The listing builds one solid part. Answer for the finished solid, in the listing's coordinates (mm). A direction names the side the tool comes from. Coordinates: 2 decimals unless noted, no trailing zeros. Loops run counter-clockwise (first coordinate to the right, second up) from the corner with the lowest first, then second, coordinate; pieces in that order, holes last. Notation, with made-up numbers: M 24,64 L 59,64 A32 cw 59,96 Z; hole C 38,-3 d10. An arc over 180 degrees is marked long. Answer as a JSON object with one key per item and string values. Group by question number.
1. Determine the mould class of faces 1 (the face through (-10, -7.2, -6)), 2 (the face through (1.325, -6.707, 6.165)), 3 (the face through (3.75, -4, 0)), 4 (the face through (-9.3, -0.1, -2.3)) for opening direction X: released by +X, released by -X, zero draft, split by the parting line, or undercut.
2. Straight lines are drawn through the part: L1, parallel to Y at x = -9.25, z = 6.75; L2, parallel to Y at x = 0.5, z = -0.75; L3, parallel to Z at x = -3.75, y = -9.5 (3 decimals). For each, find the intervals that lie inside material, in ascending order.
3. A cutting plane is placed at C-C on z = -2.5. Give the vertices of the cut face in (x, y), and give its area (3 significant figures).
4. For faces 5 (the face through (2, -0.1, -2)), 6 (the face through (-10, -7.2, 6)), determine the directions among +Z, -Z, +X, -X, +Y, -Y from which every point of the face is accessible in a straight line to the end or side of a thin tool.
5. A cutting plane is placed at A-A on y = -8.5. State how many separate pieces and enclosed holes the cut face has, and give its area (3 significant figures).
6. Given pin 1 (6 mm diameter, centred on x = -4, y = -6.5, fed in from -Z); pin 2 (0.6 mm diameter, centred on x = 0.5, z = 0, fed in from +Y); pin 3 (0.5 mm diameter, centred on x = -10.5, z = 6, fed in from -Y), each flat-ended and moving along its own axis, determine where each tip first touches the part or whether it passes through.
7. A cutting plane is placed at B-B on x = 0.75. Give the vertices of the cut face in (y, z).
from build123d import *

# Parameters (mm, degrees)
SKETCH1_W               = 15
SKETCH1_H               = 14
EXTRUDE1_DEPTH          = 7.2
SKETCH6_R               = 0.45
CUT_EXTRUDE1_DEPTH      = 0.1
CUT_EXTRUDE2_DEPTH      = 1
CUT_EXTRUDE2_DEPTH_BACK = 16
CUT_EXTRUDE3_DEPTH      = 1
CUT_EXTRUDE3_DEPTH_BACK = 15
LPATTERN2_COUNT         = 2
LPATTERN2_PITCH         = 7.5
BOSS_EXTRUDE4_START     = -1
SKETCH11_R              = 0.225
BOSS_EXTRUDE4_DEPTH     = 7.1
LPATTERN3_COUNT         = 5
LPATTERN3_PITCH         = 2.54
LPATTERN3_COUNT_DIR2    = 2
LPATTERN3_PITCH_DIR2    = 10.16


with BuildPart() as part:
    # Sketch1 → Extrude1 (new body)
    with BuildSketch(Plane(origin=(0, 0, 0), x_dir=(1, 0, 0), z_dir=(0, 1, 0))):
        with Locations((-3.75, 0)):
            Rectangle(SKETCH1_W, SKETCH1_H)
    extrude(amount=-EXTRUDE1_DEPTH)

    # Sketch6 → Cut-Extrude1 (cut)
    with BuildSketch(Plane(origin=(0, 0, 0), x_dir=(-1, 0, 0), z_dir=(0, 1, 0))):
        with Locations((-2.828914589, 5.1)):
            Circle(SKETCH6_R)
        Polygon((1.615140342, 0.645647316), (1.874984591, 3.615680666), (2.672057265, 4.346063205), (2.736318521, 4.281801948), (2.412096101, 0.575922722), (1.978755924, 0.212307139), align=None)
        Polygon((-2.08510989, 4.246446609), (-2.404999919, 0.590086851), (-2.118563171, 0.248724827), (-1.593244842, 0.689519243), (-1.335889658, 3.631102448), (-1.988382771, 4.343173729), align=None)
        Polygon((-2.751982586, -4.346963991), (-2.828914589, -4.255280001), (-2.499336567, -0.488185972), (-2.097293847, -0.150832074), (-1.707416581, -0.615469707), (-1.976986224, -3.696664829), align=None)
        Polygon((-2.591285684, -4.538475102), (-1.79792785, -3.872768836), (1.154576659, -3.872768836), (1.713170541, -4.538475102), (1.639848023, -4.6), (-2.539660165, -4.6), align=None)
        Polygon((1.560181456, -0.4), (1.954104558, -0.069459271), (1.560181456, 0.4), (-1.627135675, 0.4), (-2.021058776, 0.069459271), (-1.627135675, -0.4), align=None)
        Polygon((2.495112157, 4.523008313), (2.41812047, 4.6), (-1.7315565, 4.6), (-1.811437663, 4.520118836), (-1.151570324, 3.8), (1.706087039, 3.8), align=None)
        Polygon((1.982853172, -0.306417777), (2.30166085, -0.686357973), (1.984568022, -4.310745576), (1.904681652, -4.377778199), (1.244483112, -3.590984217), (1.496113015, -0.714841264), align=None)
    cut_extrude1 = extrude(amount=-CUT_EXTRUDE1_DEPTH, mode=Mode.SUBTRACT)

    # Sketch12 → Cut-Extrude2 (cut, two sides)
    with BuildSketch(Plane.ZY.offset(11.25)) as cut_extrude2_sk:
        Polygon((-20.043427491, -42.781711537), (-5.305, -7.2), (-4.890786438, -6.2), (4.890786438, -6.2), (5.305, -7.2), (20.043427491, -42.781711537), (20.043427491, -119.808445619), (-20.043427491, -119.808445619), align=None)
    extrude(amount=CUT_EXTRUDE2_DEPTH, mode=Mode.SUBTRACT)
    extrude(cut_extrude2_sk.sketch, amount=-CUT_EXTRUDE2_DEPTH_BACK, mode=Mode.SUBTRACT)

    # Sketch13 → Cut-Extrude3 (cut, two sides)
    with BuildSketch(Plane(origin=(0, 0, -7), x_dir=(-1, 0, 0), z_dir=(0, 0, -1))) as cut_extrude3_sk:
        Polygon((-1.555, -7.2), (-1.088692342, -6.2), (8.588692342, -6.2), (9.055, -7.2), align=None)
    extrude(amount=CUT_EXTRUDE3_DEPTH, mode=Mode.SUBTRACT)
    extrude(cut_extrude3_sk.sketch, amount=-CUT_EXTRUDE3_DEPTH_BACK, mode=Mode.SUBTRACT)

    # LPattern2: Cut-Extrude1 ×2
    with Locations(*[(-i * LPATTERN2_PITCH, 0, 0) for i in range(1, LPATTERN2_COUNT)]):
        add(cut_extrude1, mode=Mode.SUBTRACT)

    # Sketch11 → Boss-Extrude4 (add)
    with BuildSketch(Plane.XZ.offset(7.2).offset(BOSS_EXTRUDE4_START)):
        with Locations((1.33, 5.08)):
            Circle(SKETCH11_R)
    boss_extrude4 = extrude(amount=BOSS_EXTRUDE4_DEPTH)

    # LPattern3: Boss-Extrude4 5 × 2
    with Locations(*[(-i * LPATTERN3_PITCH, 0, -j * LPATTERN3_PITCH_DIR2) for i in range(LPATTERN3_COUNT) for j in range(LPATTERN3_COUNT_DIR2) if (i, j) != (0, 0)]):
        add(boss_extrude4)


solid = part.part
From the geometry:
{
 "1": {"face 1": "zero draft", "face 2": "undercut", "face 3": "released by +X", "face 4": "undercut"},
 "2": {"L1": "y = -7.2 to 0", "L2": "y = -6.2 to 0", "L3": "z = -5.305 to -4.855, 4.855 to 5.305"},
 "3": {"outline": "M -11.25,-6.2 L 3.75,-6.2 L 3.75,0 L 2.68,0 L 2.68,-0.1 L 1.87,-0.1 L 1.87,0 L -1.34,0 L -1.34,-0.1 L -2.14,-0.1 L -2.14,0 L -4.82,0 L -4.82,-0.1 L -5.63,-0.1 L -5.63,0 L -8.84,0 L -8.84,-0.1 L -9.64,-0.1 L -9.64,0 L -11.25,0 Z", "area": "92.7 mm²"},
 "4": {"face 5": "+Y", "face 6": "+Z, -Z, +X, -X, -Y"},
 "5": {"separate pieces": "10", "enclosed holes": "0", "area": "1.59 mm²"},
 "6": {"pin 1": "stops at z = -7", "pin 2": "stops at y = -0.1", "pin 3": "stops at y = -7.2"},
 "7": {"outline": "M -6.2,-7 L 0,-7 L 0,-4.6 L -0.1,-4.6 L -0.1,-3.87 L 0,-3.87 L 0,-0.4 L -0.1,-0.4 L -0.1,0.4 L 0,0.4 L 0,3.8 L -0.1,3.8 L -0.1,4.6 L 0,4.6 L 0,7 L -6.2,7 Z"}
}
